from build123d import *

# Parameters (mm, degrees)
F0_W     = 127
F0_H     = 76.2
F0_R     = 6.35
F1_DEPTH = 50.8
F2_R     = 26.547784
F3_DEPTH = 50.801


with BuildPart() as f1:
    # F0 (on Top) → F1 (new body)
    with BuildSketch(Plane.XY):
        Rectangle(F0_W, F0_H)
        with Locations((-50.8, -25.4)):
            Circle(F0_R, mode=Mode.SUBTRACT)
        with Locations((50.8, -25.4)):
            Circle(F0_R, mode=Mode.SUBTRACT)
        with Locations((-50.8, 25.4)):
            Circle(F0_R, mode=Mode.SUBTRACT)
        with Locations((50.8, 25.4)):
            Circle(F0_R, mode=Mode.SUBTRACT)
    extrude(amount=F1_DEPTH)

    # F2 (on Top) → F3 (cut, through all)
    with BuildSketch(Plane.XY):
        Circle(F2_R)
    extrude(amount=F3_DEPTH, mode=Mode.SUBTRACT)


solid = f1.part
Work out the finished part from the listing and answer in its coordinate system (mm). Give positions to 0.01 mm unless a question says otherwise; leave off trailing zeros. Order: outer loops, then holes, each group sorted by start corner. A loop starts at its lowest first (then second) coordinate and runs counter-clockwise, first axis right, second up. Notation, with made-up numbers: (-10.75, -29) -> (21.25, -29) arc R30 cw to (21.25, -3) -> close; hole circle Ø11 at (56.25, 36). An arc over 180 degrees is marked (long way). One line per item, written item: value.
Item 1: Determine the mould class of faces 1 (the cylindrical face through (56.666, -27.832, 25.044)), 2 (the flat face through (63.5, -1, 25)), 3 (the flat face through (-1, 38.1, 25)) for opening direction X: released by +X, released by -X, zero draft, split by the parting line, or undercut.
Answer sheet:
face 1: undercut
face 2: released by +X
face 3: zero draft
Item 2: Find section C-C, the plane z = 5. Give the vertices of the cut face in (x, y), plus the area to 3 significant figures.
Answer sheet:
outline: (-63.5, -38.1) -> (63.5, -38.1) -> (63.5, 38.1) -> (-63.5, 38.1) -> close; hole circle Ø12.7 at (-50.8, -25.4); hole circle Ø12.7 at (-50.8, 25.4); hole circle Ø53.1 at (0, 0); hole circle Ø12.7 at (50.8, -25.4); hole circle Ø12.7 at (50.8, 25.4)
area: 6,960 mm²
Item 3: Find section D-D, the plane x = 0. Give the vertices of the cut face in (y, z).
Answer sheet:
outline: (-38.1, 0) -> (-26.55, 0) -> (-26.55, 50.8) -> (-38.1, 50.8) -> close; (26.55, 0) -> (38.1, 0) -> (38.1, 50.8) -> (26.55, 50.8) -> close
Item 4: Straight lines are drawn through the part: probe 1 along Y at (x, z) = (-50.8, 27); probe 2 along X at (y, z) = (0, 32); probe 3 along Y at (x, z) = (0, 15). For each, find the intervals that lie inside material, in ascending order.
Answer sheet:
probe 1: -38.1 to -31.75, -19.05 to 19.05, 31.75 to 38.1
probe 2: -63.5 to -26.55, 26.55 to 63.5
probe 3: -38.1 to -26.55, 26.55 to 38.1
Item 5: Find section B-B, the plane y = 0. Give the vertices of the cut face in (x, z).
Answer sheet:
outline: (-63.5, 0) -> (-26.55, 0) -> (-26.55, 50.8) -> (-63.5, 50.8) -> close; (26.55, 0) -> (63.5, 0) -> (63.5, 50.8) -> (26.55, 50.8) -> close
Item 6: Find section A-A, the plane x = -50.8. Give the vertices of the cut face in (y, z).
Answer sheet:
outline: (-38.1, 0) -> (-31.75, 0) -> (-31.75, 50.8) -> (-38.1, 50.8) -> close; (-19.05, 0) -> (19.05, 0) -> (19.05, 50.8) -> (-19.05, 50.8) -> close; (31.75, 0) -> (38.1, 0) -> (38.1, 50.8) -> (31.75, 50.8) -> close
